Can you work these out from the drawing? Everything is in mm from the part's minimum corner. Coordinates: 2 decimals unless noted, no trailing zeros. Order: outer loops, then holes, each group sorted by start corner. A loop starts at its lowest first (then second) coordinate and runs counter-clockwise, first axis right, second up. Notation, with made-up numbers: (38.25, -33) -> (42.25, -33) arc R25 ccw to (42.25, -8) -> close; hole circle Ø7 at (-31.5, -29.75). An arc over 180 degrees is marked (long way). Answer in a Markdown table with one row per item.
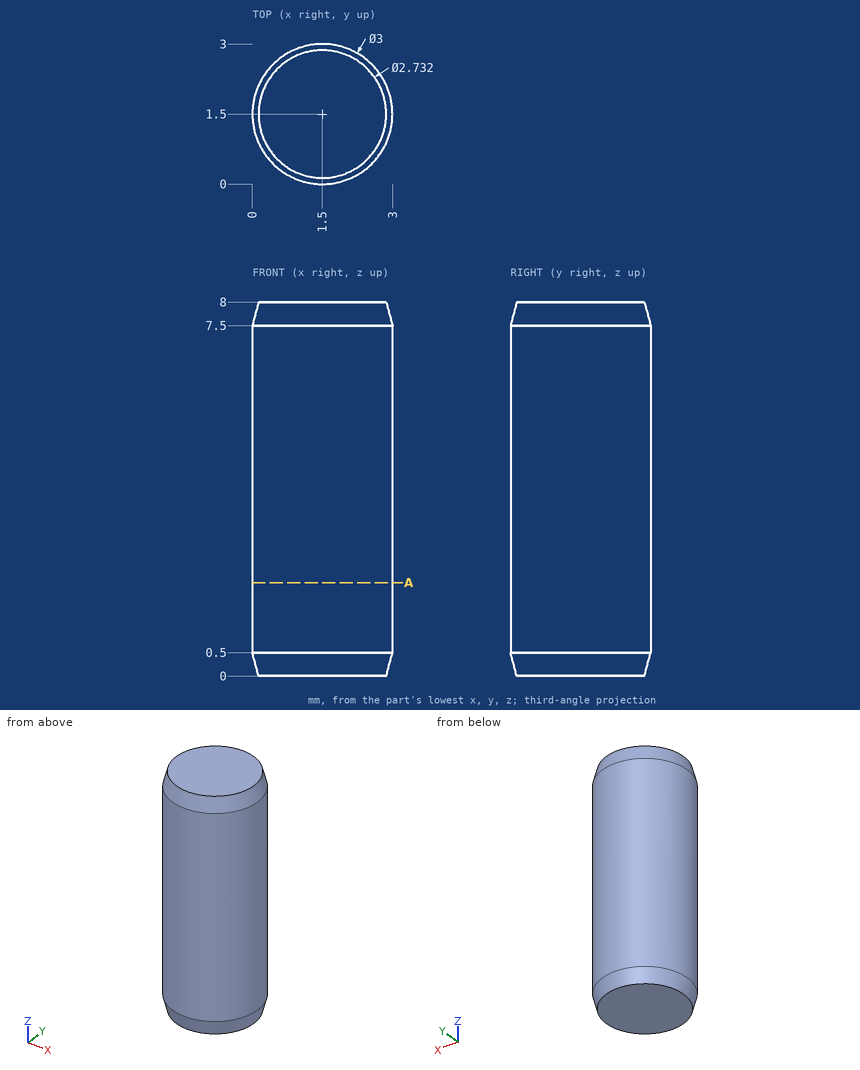
(1) I need wall thicknesses on line 1 (Y direction, x = 0.75, z = 0.75); line 2 (Y direction, x = 2.5, z = 5.75); line 3 (X direction, y = 0.25, z = 3.25). Which ranges of each line are inside material? Lowest first, please. Write a range as [from, to].
Response values:
| item | result |
|---|---|
| line 1 | [0.2, 2.8] |
| line 2 | [0.38, 2.62] |
| line 3 | [0.67, 2.33] |
(2) Suppose I cut it at A-A (z = 2). Please give me the cut outline in (x, y).
Response values:
| item | result |
|---|---|
| outline | circle Ø3 at (1.5, 1.5) |
(3) Will these pins go through, and if not, where does the flat tip stop? pin 1 Ø1.5 at (y, z) = (0.5, 6.5) entering from +X; pin 2 Ø1.5 at (x, z) = (2.5, 4) entering from +Y.
Response values:
| item | result |
|---|---|
| pin 1 | x = 2.98 |
| pin 2 | y = 2.98 |
